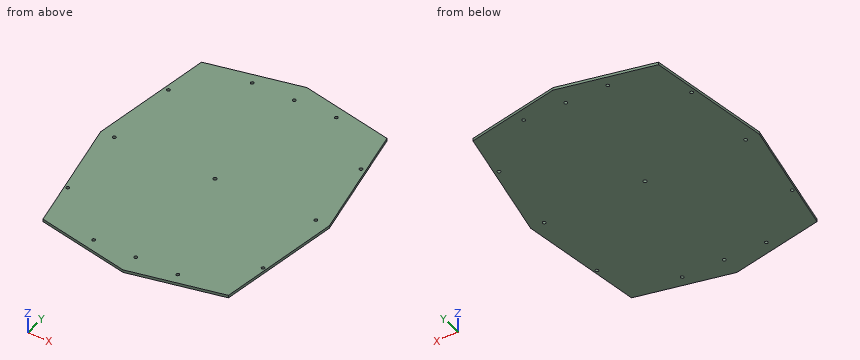
from build123d import *

# Parameters (mm, degrees)
SKETCH1_R              = 1.89865
SKETCH1_R_2            = 1.869185851
MAINBODY_DEPTH         = 3.175
F_10_32_TAPPED_HOLE1_D = 4.0386


with BuildPart() as part:
    # Sketch1 → MainBody (new body)
    with BuildSketch(Plane.XY.offset(-617.860281703)):
        Polygon((-107.5, 142.639876692), (-132.56321938, 0), (-107.5, -142.639876692), (0, -165.569938346), (107.5, -142.639876692), (132.56321938, 0), (107.5, 142.639876692), (0, 165.569938346), align=None)
        with Locations((48.75, -142.639876692)):
            Circle(SKETCH1_R, mode=Mode.SUBTRACT)
        with Locations((0, -142.639876692)):
            Circle(SKETCH1_R, mode=Mode.SUBTRACT)
        with Locations((-48.75, -142.639876692)):
            Circle(SKETCH1_R, mode=Mode.SUBTRACT)
        with Locations((-113.226895498, -89.153367391)):
            Circle(SKETCH1_R, mode=Mode.SUBTRACT)
        with Locations((-116.750007419, 0.165666821)):
            Circle(SKETCH1_R, mode=Mode.SUBTRACT)
        with Locations((-111.690160304, 89.410835528)):
            Circle(SKETCH1_R, mode=Mode.SUBTRACT)
        with Locations((111.690160304, 89.410835528)):
            Circle(SKETCH1_R, mode=Mode.SUBTRACT)
        with Locations((116.750007419, 0.165666821)):
            Circle(SKETCH1_R, mode=Mode.SUBTRACT)
        with Locations((113.226895498, -89.153367391)):
            Circle(SKETCH1_R_2, mode=Mode.SUBTRACT)
        with Locations((48.75, 142.639876692)):
            Circle(SKETCH1_R, mode=Mode.SUBTRACT)
        with Locations((0, 142.639876692)):
            Circle(SKETCH1_R, mode=Mode.SUBTRACT)
        with Locations((-48.75, 142.639876692)):
            Circle(SKETCH1_R, mode=Mode.SUBTRACT)
    extrude(amount=MAINBODY_DEPTH)

    # #10-32 Tapped Hole1 (through all)
    with Locations(Plane.XY.offset(-614.685281703)):
        with Locations((0, 0)):
            Hole(F_10_32_TAPPED_HOLE1_D / 2)


solid = part.part
Part model, mm, in its own coordinate system. Round coordinates to 2 decimals unless told otherwise and drop trailing zeros. Loops run counter-clockwise (first coordinate to the right, second up) from the corner with the lowest first, then second, coordinate; pieces in that order, holes last. Notation, with made-up numbers: (70.5, 53.5) - (91.5, 53.5) arc R15 cw to (91.5, 65.5) - close; hole circle Ø9 at (13, 54). An arc over 180 degrees is marked (long way). Answer as a JSON object with one key per item and string values.
Item 1: Band-saw the part on C-C on y = -109. List the corners of the cut face in (x, z).
Output:
{"outline": "(-113.41, -617.86) - (113.41, -617.86) - (113.41, -614.69) - (-113.41, -614.69) - close"}
Item 2: Band-saw the part on A-A on z = -616.9. State how many separate pieces and enclosed holes the cut face has, plus the area to 3 significant figures.
Output:
{"separate pieces": "1", "enclosed holes": "13", "area": "73,300 mm2"}
Item 3: Pin check, flat tips, straight feed: pin 1 (1.5 mm diameter, centred on y = -30.5, z = -616, fed in from -X); pin 2 (1 mm diameter, centred on x = 68, z = -616, fed in from -Y). Stop position of each tip, or through.
Output:
{"pin 1": "x = -127.34", "pin 2": "y = -151.17"}
Item 4: Wall check: L1, parallel to X at y = 88, z = -616; L2, parallel to Y at x = 1, z = -616.4; L3, parallel to Y at x = -48.75, z = -616.45. Give the ranges that are in metal, low to high.
Output:
{"L1": "-117.1 to -112.96, -110.42 to 110.42, 112.96 to 117.1", "L2": "-165.36 to -144.25, -141.03 to -1.75, 1.75 to 141.03, 144.25 to 165.36", "L3": "-155.17 to -144.54, -140.74 to 140.74, 144.54 to 155.17"}
Item 5: Band-saw the part on B-B on x = 81. List the corners of the cut face in (y, z), plus the area to 3 significant figures.
Output:
{"outline": "(-148.29, -617.86) - (148.29, -617.86) - (148.29, -614.69) - (-148.29, -614.69) - close", "area": "942 mm2"}
